Here's the drawing with two shaded views (mm, measured from the low corner). I have some questions. Give positions to 0.01 mm unless a question says otherwise; leave off trailing zeros. Write each loop counter-clockwise with the first axis right and the second up, starting at its lowest first coordinate (ties: lowest second). Pieces come first, ordered by that corner, then holes.
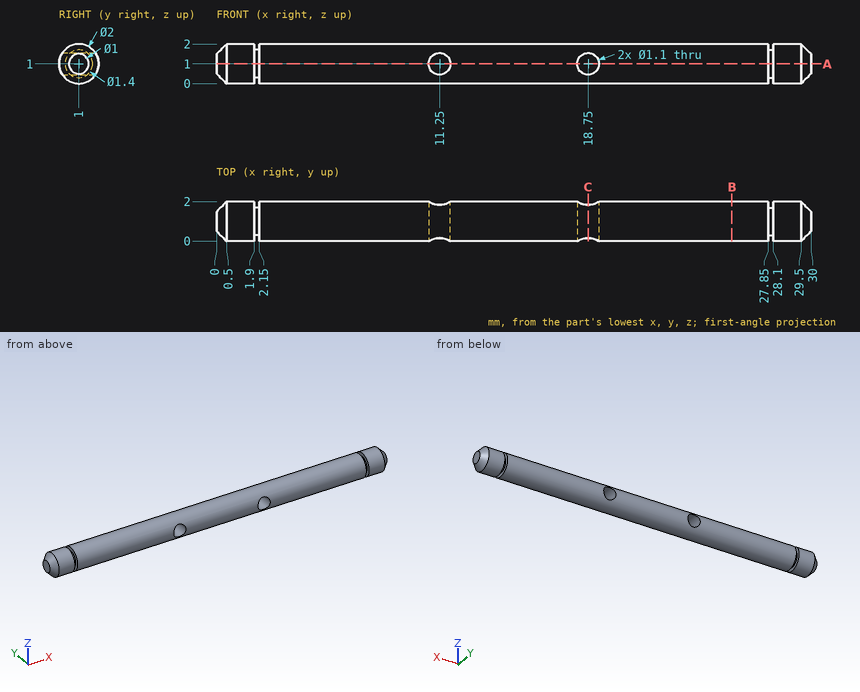
1) Suppose I cut it at C-C on x = 18.75. Write out the boundary of the cut face in (y, z).
Values follow:
outline: (0.16, 0.45) arc R1 ccw to (1.84, 0.45) - close; (0.16, 1.55) - (1.84, 1.55) arc R1 ccw to start
2) Suppose I cut it at A-A on z = 1. State how many separate pieces and enclosed holes the cut face has, plus the area to 3 significant figures.
Values follow:
separate pieces: 3
enclosed holes: 0
area: 54.8 mm2
3) Suppose I cut it at B-B on x = 26. Write out the boundary of the cut face in (y, z), plus the area to 3 significant figures.
Values follow:
outline: circle Ø2 at (1, 1)
area: 3.14 mm2
4) Please list where these lines run through material, in increasing order: L1, parallel to X at y = 1.15, z = 1.75; L2, parallel to X at y = 0.7, z = 1.4; L3, parallel to Z at x = 11.25, y = 1.1.
Values follow:
L1: x = 0.26 to 1.9, 2.15 to 27.85, 28.1 to 29.74
L2: x = 0 to 10.87, 11.63 to 18.37, 19.13 to 30
L3: z = 0.01 to 0.45, 1.55 to 1.99
